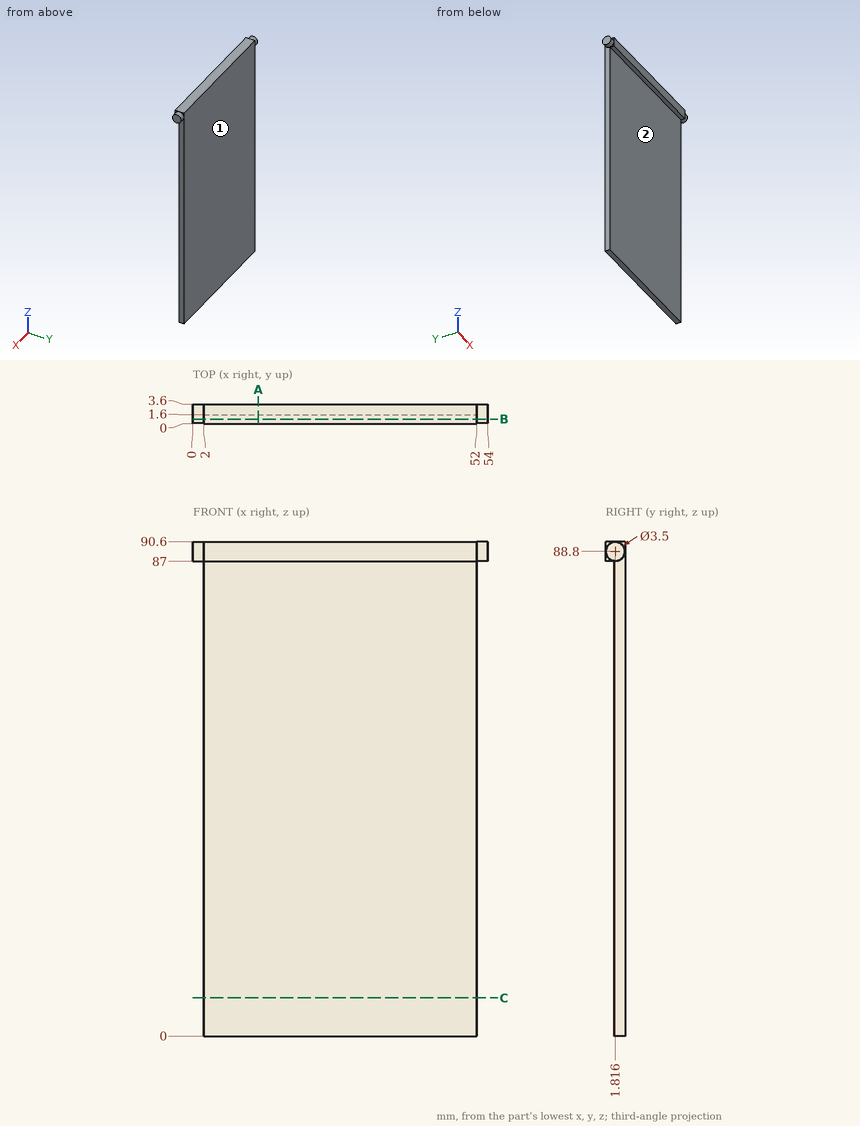
For this review, use the dimensioned drawing (mm, ordinates from the lowest corner) and the shaded views. A direction names the side the tool comes from. Give positions to 0.01 mm unless a question says otherwise; leave off trailing zeros. Write each loop counter-clockwise with the first axis right and the second up, starting at its lowest first coordinate (ties: lowest second). Pieces come first, ordered by that corner, then holes. Notation, with made-up numbers: M 31.25,88 L 90.25,88 A8 cw 90.25,93 Z; hole C -29.5,-37 d8. An arc over 180 degrees is marked long. Answer as a JSON object with one key per item and string values. Group by question number.
1) Tool access review of the marked faces 1 and 2: name each direction out of +Z, -Z, +X, -X, +Y, -Y from which nothing blocks a thin tool from reaching the whole face with its end or side.
2) We need section C-C (z = 7). Give the boundary of the cut face in (x, y), and give its area (3 significant figures).
3) We need section A-A (x = 12). Give the boundary of the cut face in (y, z).
4) For line 1 along X through (y, z) = (2.4, 11.5); line 2 along Y through (x, z) = (29, 58.5); line 3 along Z through (x, y) = (25, 1.3), list the stretches that pass through material, from the lowest coordinate up.
5) Clearance check with flat-ended pins moving along their axes: pin 1 Ø1.8 at (y, z) = (1.5, 45) entering from +X; pin 2 Ø15 at (x, z) = (39.5, 51) entering from -Y; pin 3 Ø0.8 at (x, y) = (33.5, 1) entering from -Z. State where each tip first meets the part, or that it passes through.
6) We need section B-B (y = 0.85). Give the boundary of the cut face in (x, z), and give its area (3 significant figures).
Answer key:
{
 "1": {"face 1": "+Z, -Z, +X, -X, +Y", "face 2": "-Z, +X, -X, -Y"},
 "2": {"outline": "M 2,1.6 L 52,1.6 L 52,3.6 L 2,3.6 Z", "area": "100 mm²"},
 "3": {"outline": "M 0,87 L 1.6,87 L 1.6,0 L 3.6,0 L 3.6,90.6 L 0,90.6 Z"},
 "4": {"line 1": "x = 2 to 52", "line 2": "y = 1.6 to 3.6", "line 3": "z = 87 to 90.6"},
 "5": {"pin 1": "stops at x = 52", "pin 2": "stops at y = 1.6", "pin 3": "stops at z = 87"},
 "6": {"outline": "M 0,87.34 L 2,87.34 L 2,87 L 52,87 L 52,87.34 L 54,87.34 L 54,90.26 L 52,90.26 L 52,90.6 L 2,90.6 L 2,90.26 L 0,90.26 Z", "area": "192 mm²"}
}
